Geometry: final body of the model. Coordinates: model frame, mm. A direction names the side the tool comes from. Give positions to 0.01 mm unless a question says otherwise; leave off trailing zeros. Loops run counter-clockwise (first coordinate to the right, second up) from the corner with the lowest first, then second, coordinate; pieces in that order, holes last. Notation, with made-up numbers: M -15.5,21.5 L 37.5,21.5 A16 ccw 37.5,33.5 Z; hole C 88,66 d4. An arc over 180 degrees is marked long. One line per question, with ' | ' between items. Start each with the question number.
Autodesk Fusion 360 part; units mm, degrees
sketch "Sketch1" plane through (0, 0, 0) normal (0, 1, 0) x (1, 0, 0)
  line L0 (0, 0) -> (85, 0)
  line L1 (85, 0) -> (85, -33)
  line L2 (85, -33) -> (0, -33)
  line L3 (0, -33) -> (0, 0)
  line L4 (0, 0) -> (85, 0)
  line L5 (85, 0) -> (85, -20)
  line L6 (85, -20) -> (0, -20)
  line L7 (0, -20) -> (0, 0)
  dimension "d1" = 85
  dimension "d2" = 33
  dimension "d3" = 20
extrude "Extrude1" add sketch "Sketch1" along normal blind 5
extrude "Extrude2" add sketch "Sketch1" against normal blind 11 contours L1 L2 L3 L6
sketch "Sketch2" plane through (0, -11, 0) normal (0, -1, 0) x (1, 0, 0)
  line L0 (85, 20) -> (85, 33)
  line L1 (85, 33) -> (0, 33)
  line L2 (0, 33) -> (0, 20)
  line L3 (0, 20) -> (85, 20)
  line L4 (0, 33) -> (15, 33)
  line L5 (15, 33) -> (15, 20)
  line L6 (15, 20) -> (0, 20)
  line L7 (0, 20) -> (0, 33)
  line L8 (85, 33) -> (70, 33)
  line L9 (70, 33) -> (70, 20)
  line L10 (70, 20) -> (85, 20)
  line L11 (85, 20) -> (85, 33)
  dimension "d8" = 15
extrude "Extrude3" cut sketch "Sketch2" against normal blind 11 contours L1 L3 L5 L9
sketch "Sketch3" plane through (0, 5, 0) normal (0, 1, 0) x (-1, 0, 0)
  line L0 (0, 0) -> (0, 33)
  line L1 (0, 33) -> (-85, 33)
  line L2 (-85, 33) -> (-85, 0)
  line L3 (-85, 0) -> (0, 0)
  line L4 (-85, 0) -> (-95, 0)
  line L5 (-95, 0) -> (-95, 33)
  line L6 (-95, 33) -> (-85, 33)
  line L7 (-85, 33) -> (-85, 0)
  circle A0 centre (-90, 16.5) radius 2.75 construction
  line L8 (-95, 16.5) -> (-85, 16.5) construction
  line L9 (-42.5, 0) -> (-42.5, 33) construction
  line L10 (0, 0) -> (10, 0)
  line L11 (10, 0) -> (10, 33)
  line L12 (10, 33) -> (0, 33)
  line L13 (0, 33) -> (0, 0)
  circle A1 centre (5, 16.5) radius 2.75 construction
  dimension "d11" = 10
  dimension "d12" = 5.5
extrude "Extrude4" add sketch "Sketch3" against normal blind 5 contours L0 L10 L11 L12 L13 | L2 L4 L5 L6 L7
sketch "Sketch4" plane through (-10, 0, 0) normal (-1, 0, 0) x (0, 0, 1)
  line L0 (33, 5) -> (0, 5)
  line L1 (0, 5) -> (0, 0)
  line L2 (0, 0) -> (33, 0)
  line L3 (33, 0) -> (33, 5)
  line L4 (33, 5) -> (-5.1734, 27.0394)
  line L5 (0, 5) -> (0, 0)
  line L6 (0, 0) -> (-15.5885, 9)
  line L7 (-15.5885, 9) -> (-5.1734, 27.0394)
  dimension "d17" = 30
  dimension "d50" = 18
extrude "Extrude5" add sketch "Sketch4" against normal blind 105 contours L0 L1 L4 L5 L6 L7
sketch "Sketch5" plane through (95, 0, 0) normal (1, 0, 0) x (0, 0, -1)
  line L0 (-33, 5) -> (-33, 0)
  line L1 (-33, 0) -> (0, 0)
  line L2 (0, 0) -> (15.5885, 9)
  line L3 (15.5885, 9) -> (5.1734, 27.0394)
  line L4 (5.1734, 27.0394) -> (-33, 5)
  line L5 (14.0885, 11.5981) -> (5.1734, 27.0394)
  line L6 (5.1734, 27.0394) -> (-7.817, 19.5394)
  line L7 (-7.817, 19.5394) -> (1.0981, 4.0981)
  line L8 (1.0981, 4.0981) -> (14.0885, 11.5981)
  line L9 (0, 0) -> (2.5981, 1.5)
  line L10 (1.0981, 4.0981) -> (2.5981, 1.5) construction
  dimension "d48" = 3
  dimension "d51" = 3
extrude "Extrude7" cut sketch "Sketch5" against normal blind 140 contours L3 L4 L5 L6 L7 L8
sketch "Sketch9" plane through (0, 2.5981, 1.5) normal (0, 0.866, 0.5) x (1, 0, 0)
  line L0 (-10, 18) -> (-10, 3)
  line L1 (-10, 3) -> (95, 3)
  line L2 (95, 3) -> (95, 18)
  line L3 (95, 18) -> (-10, 18)
  circle A0 centre (10, 10.5) radius 1.75
  circle A1 centre (75, 10.5) radius 1.75
  dimension "d55" = 3.5
  dimension "d56" = 3.5
  dimension "d57" = 7.5
  dimension "d58" = 20
  dimension "d59" = 20
extrude "Extrude11" cut sketch "Sketch9" along direction (0, -0.5, -0.866025) blind 16 contours A0 | A1
sketch "Sketch8" plane through (0, 0, 0) normal (0, -1, 0) x (1, 0, 0)
  line L0 (85, 20) -> (70, 20)
  line L1 (70, 20) -> (70, 33)
  line L2 (70, 33) -> (15, 33)
  line L3 (15, 33) -> (15, 20)
  line L4 (15, 20) -> (0, 20)
  line L5 (0, 20) -> (0, 33)
  line L6 (0, 33) -> (-10, 33)
  line L7 (-10, 33) -> (-10, 0)
  line L8 (95, 0) -> (95, 33)
  line L9 (95, 33) -> (85, 33)
  line L10 (85, 33) -> (85, 20)
  arc A0 (30.5, 33) -> (54.5, 33) centre (42.5, 37) ccw
  line L11 (42.5, 33) -> (54.5, 33)
  line L12 (42.5, 33) -> (30.5, 33)
  line L13 (42.5, 37) -> (42.5, 33) construction
  line L14 (-10, 0) -> (95, 0)
  dimension "d44" = 12
  dimension "d45" = 4
extrude "Extrude10" cut sketch "Sketch8" against normal blind 25 contours L2 A0 L11 L12
fillet "Fillet2" radius 15 1 edges at (42.5, 19.5394, 7.817)
sketch "Sketch10" plane through (0, 0, 0) normal (0, -1, 0) x (1, 0, 0)
  arc A0 (30.5, 33) -> (54.5, 33) centre (42.5, 37) ccw
  line L0 (30.5, 33) -> (15, 33)
  line L1 (15, 33) -> (15, 20)
  line L2 (15, 20) -> (0, 20)
  line L3 (0, 20) -> (0, 33)
  line L4 (0, 33) -> (-10, 33)
  line L5 (-10, 33) -> (-10, 0)
  line L6 (-10, 0) -> (95, 0)
  line L7 (95, 0) -> (95, 33)
  line L8 (95, 33) -> (85, 33)
  line L9 (85, 33) -> (85, 20)
  line L10 (85, 20) -> (70, 20)
  line L11 (70, 20) -> (70, 33)
  line L12 (70, 33) -> (54.5, 33)
  circle A1 centre (-5, 18) radius 2.75
  circle A2 centre (90, 18) radius 2.75
  dimension "d63" = 5.5
  dimension "d64" = 5.5
  dimension "d65" = 5
  dimension "d66" = 5
  dimension "d67" = 15
extrude "Extrude12" cut sketch "Sketch10" against normal blind 25 contours A1 | A2
Q1. Set-up query: faces 4 (the flat face through (85, -5, 26)), 5 (the flat face through (78, -5, 20)), 6 (the flat face through (0, -5, 27)). Return all of +Z, -Z, +X, -X, +Y, -Y with unobstructed straight access to the full face (end or side cutting, diameter ignored); none if empty.
Q2. Section C-C, the plane x = 66.5. Output: boundary loops of the cut face in (y, z), plus the area to 3 significant figures.
Q3. Section B-B, the plane x = -5. Output: boundary loops of the cut face in (y, z).
Q4. Material intervals for L1, parallel to X at y = 9.25, z = 18; L2, parallel to Z at x = -5, y = 9; L3, parallel to Z at x = -5, y = 10.5, sorted ascending.
Q5. Draft query along Z for faces 1 (the flat face through (43.24, 5.34, -0.38)), 2 (the cylindrical face through (42.279, 3.822, 24.353)), 3 (the flat face through (7, -11, 26)). Return one class per face: released by +Z, released by -Z, zero draft, split by the parting line, or undercut.
Q6. Section A-A, the plane z = 26.5. Output: boundary loops of the cut face in (x, y), plus the area to 3 significant figures.
Q7. Contact query for flat-ended pins moving along their axis: pin 1 (5.5 mm diameter, centred on y = -6, z = 29, fed in from -X); pin 2 (5.5 mm diameter, centred on y = -8, z = 24, fed in from +X); pin 3 (6.5 mm diameter, centred on x = 90, z = 18, fed in from +Y); pin 4 (8 mm diameter, centred on y = -1.5, z = 4.5, fed in from -X). Output: stop coordinate, or through.
Q8. Section D-D, the plane z = 18. Output: boundary loops of the cut face in (x, y).
Model answer:
1) face 4: +Z, -Z, +X, -Y | face 5: -Z, +X, -X, -Y | face 6: +Z, -Z, -X, -Y
2) outline: M 0,0 L 9,-15.59 L 11.6,-14.09 L 4.1,-1.1 L 6.55,0.32 A15 ccw 12.04,20.81 L 5,33 L 0,33 Z | area: 413 mm^2
3) outline: M 0,0 L 9,-15.59 L 11.6,-14.09 L 4.1,-1.1 L 6.55,0.32 A15 ccw 13.92,15.25 L 0,15.25 Z; M 0,20.75 L 12.07,20.75 A15 ccw 12.04,20.81 L 5,33 L 0,33 Z
4) L1: x = -10 to -7.75, -2.25 to 87.25, 92.75 to 95 | L2: z = -15.59 to -9.59, 2.08 to 15.25, 20.75 to 26.07 | L3: z = -14.72 to -12.19, 3.62 to 15.25, 20.75 to 23.47
5) face 1: undercut | face 2: released by +Z | face 3: zero draft
6) outline: M -10,0 L 0,0 L 0,-11 L 15,-11 L 15,0 L 35.45,0 L 35.45,8.75 L -10,8.75 Z; M 49.55,0 L 70,0 L 70,-11 L 85,-11 L 85,0 L 95,0 L 95,8.75 L 49.55,8.75 Z | area: 1,130 mm^2
7) pin 1: stops at x = 0 | pin 2: stops at x = 85 | pin 3: stops at y = 13.98 | pin 4: stops at x = -10
8) outline: M -10,0 L -7.75,0 L -7.75,13.3 L -10,13.3 Z; M -2.25,0 L 87.25,0 L 87.25,13.3 L -2.25,13.3 Z; M 92.75,0 L 95,0 L 95,13.3 L 92.75,13.3 Z
